from build123d import *
from build123d.topology import SkipClean

# Parameters (mm, degrees)
BOSS_EXTRU_1_DEPTH      = 40
ESQUISSE2_W             = 2
ESQUISSE2_H             = 40
BOSS_EXTRU_2_DEPTH      = 12.5
BOSS_EXTRU_4_START      = -2
ESQUISSE4_R             = 4
BOSS_EXTRU_4_DEPTH      = 2
ESQUISSE5_R             = 0.5
ENL_V_MAT_EXTRU_1_DEPTH = 45.949972191
BOSS_EXTRU_13_DEPTH     = 40
BOSS_EXTRU_14_START     = 38
BOSS_EXTRU_14_DEPTH     = 38
CONG_1_R                = 1
ESQUISSE10_R            = 1.75
ENL_V_MAT_EXTRU_2_DEPTH = 54.247065647


with BuildPart() as part:
    # Esquisse1 → Boss.-Extru.1 (new body)
    with BuildSketch(Plane.XY):
        with BuildLine():
            ThreePointArc((-12.5, 0), (0, 12.5), (12.5, 0))
            Line((12.5, 0), (14.5, 0))
            ThreePointArc((14.5, 0), (0, 14.5), (-14.5, 0))
            Line((-14.5, 0), (-12.5, 0))
        make_face()
    extrude(amount=BOSS_EXTRU_1_DEPTH)

    # Esquisse2 → Boss.-Extru.2 (add)
    with BuildSketch(Plane.XZ):
        with Locations((-13.5, 20)):
            Rectangle(ESQUISSE2_W, ESQUISSE2_H)
        with Locations((13.5, 20)):
            Rectangle(ESQUISSE2_W, ESQUISSE2_H)
    extrude(amount=BOSS_EXTRU_2_DEPTH)

    # Esquisse4 → Boss.-Extru.4 (add)
    with BuildSketch(Plane.XY.offset(40).offset(BOSS_EXTRU_4_START)):
        with BuildLine():
            Line((-12.5, 0), (-12.5, -12.5))
            Line((-12.5, -12.5), (12.5, -12.5))
            Line((12.5, -12.5), (12.5, 0))
            ThreePointArc((12.5, 0), (0, 12.5), (-12.5, 0))
        make_face()
        Circle(ESQUISSE4_R, mode=Mode.SUBTRACT)
    extrude(amount=BOSS_EXTRU_4_DEPTH)

    # Esquisse5 → Enlèv. mat.-Extru.1 (cut, through all)
    with BuildSketch(Plane.XY.offset(40)):
        with Locations((0, -8)):
            Circle(ESQUISSE5_R)
        with Locations((0, 8)):
            Circle(ESQUISSE5_R)
    extrude(amount=-ENL_V_MAT_EXTRU_1_DEPTH, mode=Mode.SUBTRACT)

    # Esquisse8 → Boss.-Extru.13 (add)
    with BuildSketch(Plane.XY.offset(40)):
        Polygon((-14.5, -12.5), (-22.5, -12.5), (-22.5, -14.5), (22.5, -14.5), (22.5, -12.5), (14.5, -12.5), align=None)
    extrude(amount=-BOSS_EXTRU_13_DEPTH)

    # Esquisse9 → Boss.-Extru.14 (add)
    with SkipClean():  # the faces are left unmerged after this step: merging them gives an invalid solid
        with BuildSketch(Plane(origin=(0, 0, 38), x_dir=(-1, 0, 0), z_dir=(0, 0, -1)).offset(BOSS_EXTRU_14_START)):
            with BuildLine():
                Line((-12.5, 0), (-12.5, -12.5))
                Line((-12.5, -12.5), (-3e-08, -12.5))
                ThreePointArc((-3e-08, -12.5), (-8.838834775, -8.838834754), (-12.5, 0))
            make_face()
            with BuildLine():
                ThreePointArc((12.5, 0), (8.838834754, -8.838834775), (-3e-08, -12.5))
                Line((-3e-08, -12.5), (12.5, -12.5))
                Line((12.5, -12.5), (12.5, 0))
            make_face()
        extrude(amount=-BOSS_EXTRU_14_DEPTH)

    # Congé1
    cong_1_edges = [part.edges().sort_by_distance(p)[0] for p in [
        (-14.5, -12.5, 20),
        (14.5, -12.5, 20),
        (-22.5, -12.5, 20),
        (22.5, -12.5, 20),
    ]]
    fillet(cong_1_edges, radius=CONG_1_R)

    # Esquisse10 → Enlèv. mat.-Extru.2 (cut, through all)
    with SkipClean():  # the faces are left unmerged after this step: merging them gives an invalid solid
        with BuildSketch(Plane(origin=(0, -12.5, 0), x_dir=(1, 0, 0), z_dir=(0, 1, 0))):
            with Locations(Location((-18.5, -10, 0), (0, 0, 180))):
                Circle(ESQUISSE10_R)
            with Locations(Location((-18.5, -30, 0), (0, 0, 180))):
                Circle(ESQUISSE10_R)
            with Locations(Location((18.5, -30, 0), (0, 0, 180))):
                Circle(ESQUISSE10_R)
            with Locations(Location((18.5, -10, 0), (0, 0, 180))):
                Circle(ESQUISSE10_R)
        extrude(amount=-ENL_V_MAT_EXTRU_2_DEPTH, mode=Mode.SUBTRACT)


solid = part.part
Model file for the job. Use its own axes, mm. A direction names the side the tool comes from. Give positions to 0.01 mm unless a question says otherwise; leave off trailing zeros. Order: outer loops, then holes, each group sorted by start corner. A loop starts at its lowest first (then second) coordinate and runs counter-clockwise, first axis right, second up. Notation, with made-up numbers: (8, 65.5) - (35, 65.5) arc R28 cw to (35, 87.5) - close; hole circle Ø4 at (-24.5, 12). An arc over 180 degrees is marked (long way). Return JSON: item names as keys, results as strings.
1) Probe line 1 (Z direction, x = 18.5, y = -13.85); line 2 (Y direction, x = 0, z = 39.15); line 3 (X direction, y = -10, z = 26.5). List the from-to ranges inside material, lowest first. Write a range as from..to.
Geometry says:
{"line 1": "0..8.25, 11.75..28.25, 31.75..40", "line 2": "-14.5..-8.5, -7.5..-4, 4..7.5, 8.5..14.5", "line 3": "-14.5..-7.5, 7.5..14.5"}
2) Flat gauge pins, fed straight in: P1, Ø1, axis at y = -7, z = 4.5, coming from the +X side; P2, Ø2, axis at x = -11, z = 17, coming from the +Y side; P3, Ø6, axis at y = -6, z = 21.5, coming from the -X side. Where does each tip first touch, or does it go through?
Geometry says:
{"P1": "x = 14.5", "P2": "y = 10.5", "P3": "x = -14.5"}
3) Pull direction Y, two halves, no side cores. Call faces 4 (the flat face through (19, -12.5, 20)), 5 (the flat face through (0, -6, 40)), 6 (the cylindrical face through (-0.867, -3.905, 38.986)): pulls with the +Y half, pulls with the -Y half, needs draft (parallel to the pull), parting line crosses it, or undercut.
Geometry says:
{"face 4": "pulls with the +Y half", "face 5": "needs draft", "face 6": "undercut"}
4) Cut at C-C, the plane z = 24. Give the cut face in (x, y), plus the area to 3 significant figures.
Geometry says:
{"outline": "(-22.5, -14.5) - (22.5, -14.5) - (22.5, -13.5) arc R1 ccw to (21.5, -12.5) - (15.5, -12.5) arc R1 cw to (14.5, -11.5) - (14.5, 0) arc R14.5 ccw to (-14.5, 0) - (-14.5, -11.5) arc R1 cw to (-15.5, -12.5) - (-21.5, -12.5) arc R1 ccw to (-22.5, -13.5) - close; hole circle Ø25 at (0, 0)", "area": "292 mm²"}
5) 3-axis set-ups, long thin cutter, end or side, ignore diameter. For faces 1 (the flat face through (14.5, -6, 20)), 2 (the flat face through (-3, 3, 38)), 3 (the flat face through (-18, -12.5, 20)): which of +Z, -Z, +X, -X, +Y, -Y reach the whole face in a straight line?
Geometry says:
{"face 1": "+Z, -Z, +X, +Y", "face 2": "-Z", "face 3": "+Z, -Z, -X, +Y"}
6) Cut at A-A, the plane z = 10. Give the cut face in (x, y).
Geometry says:
{"outline": "(-22.5, -14.5) - (-20.25, -14.5) - (-20.25, -12.5) - (-21.5, -12.5) arc R1 ccw to (-22.5, -13.5) - close; (-16.75, -14.5) - (16.75, -14.5) - (16.75, -12.5) - (15.5, -12.5) arc R1 cw to (14.5, -11.5) - (14.5, 0) arc R14.5 ccw to (-14.5, 0) - (-14.5, -11.5) arc R1 cw to (-15.5, -12.5) - (-16.75, -12.5) - close; (20.25, -14.5) - (22.5, -14.5) - (22.5, -13.5) arc R1 ccw to (21.5, -12.5) - (20.25, -12.5) - close; hole circle Ø25 at (0, 0)"}
7) Cut at D-D, the plane x = -10. Give the cut face in (y, z).
Geometry says:
{"outline": "(-14.5, 0) - (-7.5, 0) - (-7.5, 38) - (7.5, 38) - (7.5, 0) - (10.5, 0) - (10.5, 40) - (-14.5, 40) - close"}
8) Cut at B-B, the plane x = 18.5. Give the cut face in (y, z).
Geometry says:
{"outline": "(-14.5, 0) - (-12.5, 0) - (-12.5, 8.25) - (-14.5, 8.25) - close; (-14.5, 11.75) - (-12.5, 11.75) - (-12.5, 28.25) - (-14.5, 28.25) - close; (-14.5, 31.75) - (-12.5, 31.75) - (-12.5, 40) - (-14.5, 40) - close"}
